```python
from build123d import *
from OCP.BRepFilletAPI import BRepFilletAPI_MakeChamfer

# Parameters (mm, degrees)
SKETCH1_W           = 20.32
SKETCH1_H           = 11.938
BOSS_EXTRUDE1_DEPTH = 10.4648
SKETCH2_W           = 20.828
SKETCH2_H           = 14.8336
BOSS_EXTRUDE2_DEPTH = 2.1844
CHAMFER1_SIZE       = 0.635
CHAMFER1_SIZE2      = 2.644965354
BOSS_EXTRUDE3_DEPTH = 4.8768


with BuildPart() as part:
    # Sketch1 → Boss-Extrude1 (new body)
    with BuildSketch(Plane(origin=(0, 0, 0), x_dir=(1, 0, 0), z_dir=(0, 1, 0))):
        Rectangle(SKETCH1_W, SKETCH1_H)
    extrude(amount=-BOSS_EXTRUDE1_DEPTH)

    # Sketch2 → Boss-Extrude2 (add)
    with BuildSketch(Plane(origin=(0, 0, 0), x_dir=(1, 0, 0), z_dir=(0, 1, 0))):
        Rectangle(SKETCH2_W, SKETCH2_H)
    extrude(amount=BOSS_EXTRUDE2_DEPTH)

    # Chamfer1: one chamfer whose edges measure the first distance from different faces: ONE call of the kernel's chamfer builder (chamfer() names one face for all edges)
    chamfer1_edges_1 = [part.edges().sort_by_distance(p)[0] for p in [
        (10.414, 2.1844, 0),
    ]]
    chamfer1_side_1 = [part.faces().sort_by_distance(p)[0] for p in [
        (10.414, 1.0922, 0),
    ]]
    chamfer1_edges_2 = [part.edges().sort_by_distance(p)[0] for p in [
        (0, 2.1844, -7.4168),
    ]]
    chamfer1_side_2 = [part.faces().sort_by_distance(p)[0] for p in [
        (0, 1.0922, -7.4168),
    ]]
    chamfer1_edges_3 = [part.edges().sort_by_distance(p)[0] for p in [
        (-10.414, 2.1844, 0),
    ]]
    chamfer1_side_3 = [part.faces().sort_by_distance(p)[0] for p in [
        (-10.414, 1.0922, 0),
    ]]
    chamfer1_edges_4 = [part.edges().sort_by_distance(p)[0] for p in [
        (0, 2.1844, 7.4168),
    ]]
    chamfer1_side_4 = [part.faces().sort_by_distance(p)[0] for p in [
        (0, 1.0922, 7.4168),
    ]]
    chamfer1 = BRepFilletAPI_MakeChamfer(part.part.solid().wrapped)
    for e in chamfer1_edges_1:
        chamfer1.Add(CHAMFER1_SIZE, CHAMFER1_SIZE2, e.wrapped, chamfer1_side_1[0].wrapped)  # the first distance lies on this face
    for e in chamfer1_edges_2:
        chamfer1.Add(CHAMFER1_SIZE, CHAMFER1_SIZE2, e.wrapped, chamfer1_side_2[0].wrapped)  # the first distance lies on this face
    for e in chamfer1_edges_3:
        chamfer1.Add(CHAMFER1_SIZE, CHAMFER1_SIZE2, e.wrapped, chamfer1_side_3[0].wrapped)  # the first distance lies on this face
    for e in chamfer1_edges_4:
        chamfer1.Add(CHAMFER1_SIZE, CHAMFER1_SIZE2, e.wrapped, chamfer1_side_4[0].wrapped)  # the first distance lies on this face
    add(Compound.cast(chamfer1.Shape()), mode=Mode.REPLACE)

    # Sketch11 → Boss-Extrude3 (add, symmetric)
    with BuildSketch(Plane.XY):
        with BuildLine():
            Line((-7.769034646, 2.1844), (7.769034646, 2.1844))
            add(Edge.make_bspline(
                [(3.914965354, 6.0198), (6.076533794, 4.336461904), (7.769034646, 2.1844)],
                knots=[0, 0, 0, 1, 1, 1], degree=2))
            add(Edge.make_bspline(
                [(-7.769034646, 2.1844), (-1.382026132, 2.477514442), (3.914965354, 6.0198)],
                knots=[0, 0, 0, 1, 1, 1], degree=2))
        make_face()
    extrude(amount=BOSS_EXTRUDE3_DEPTH, both=True)


solid = part.part
```
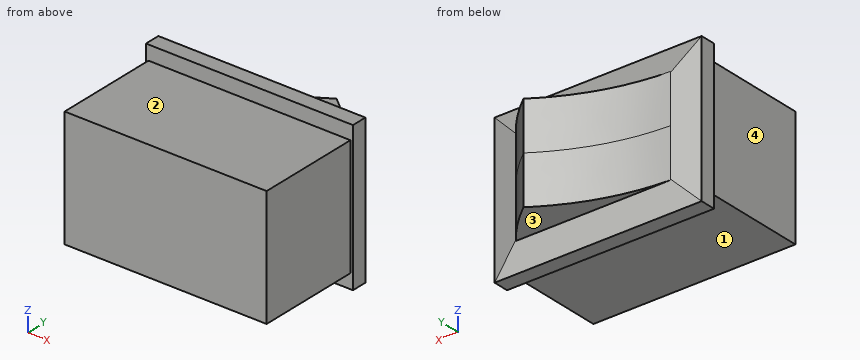
Input: part model. Units: mm. Frame: model coordinates. Face numbers are marked on the shaded views. A direction names the side the tool comes from. Give positions to 0.01 mm unless a question says otherwise; leave off trailing zeros. Order: outer loops, then holes, each group sorted by start corner. A loop starts at its lowest first (then second) coordinate and runs counter-clockwise, first axis right, second up. Notation, with made-up numbers: (66.5, 46.25) -> (81.5, 46.25) arc R19 cw to (81.5, 53.25) -> close; hole circle Ø8 at (4, 26.25). An arc over 180 degrees is marked (long way). Write each question's results on one line, items separated by ' | '. Start each with the question number.
Item 1: Line query: line 1 (Z direction, x = 7, y = -1); line 2 (X direction, y = -2.5, z = 4.25); line 3 (Y direction, x = -4, z = 5.75). Output: solid intervals per line, ascending.
Item 2: Contact query for flat-ended pins moving along their axis: P1, Ø3, axis at y = -7, z = -0.5, coming from the -X side; P2, Ø2, axis at x = 1.5, y = -8, coming from the +Z side; P3, Ø3, axis at y = -4, z = 2.5, coming from the +X side. Output: stop coordinate, or through.
Item 3: Set-up query: the marked faces 1, 2, 3 and 4. Return all of +Z, -Z, +X, -X, +Y, -Y with unobstructed straight access to the full face (end or side cutting, diameter ignored); none if empty.
Item 4: Cut plane B-B on y = -1. Return the cut outline in (x, z).
Item 5: Cut plane A-A on z = 6.5. Return the cut outline in (x, y).
Established:
1) line 1: -5.97 to 5.97 | line 2: -10.16 to 10.16 | line 3: -10.46 to 1.95
2) P1: x = -10.16 | P2: z = 5.97 | P3: x = 10.16
3) face 1: -Z, +X, -X, -Y | face 2: +Z, +X, -X, -Y | face 3: -Z, +X, -X, +Y | face 4: +Z, -Z, -X, -Y
4) outline: (-10.16, -5.97) -> (10.16, -5.97) -> (10.16, 5.97) -> (-10.16, 5.97) -> close
5) outline: (-10.41, 0) -> (10.41, 0) -> (10.41, 1.55) -> (9.5, 1.77) -> (-9.5, 1.77) -> (-10.41, 1.55) -> close
